Part model, mm, in its own coordinate system. Face numbers are marked on the shaded views. Coordinates: 2 decimals unless noted, no trailing zeros. Loops run counter-clockwise (first coordinate to the right, second up) from the corner with the lowest first, then second, coordinate; pieces in that order, holes last. Notation, with made-up numbers: (41.25, 31) -> (72.25, 31) arc R21 ccw to (72.25, 48) -> close; hole circle Ø2 at (-32, 74). An arc over 180 degrees is marked (long way). Use one line per item in the form item = value. Start each with the question number.
(1) Band-saw the part on B-B on x = -3.75. Give the cut face in (y, z) (3 decimals).
(2) Band-saw the part on A-A on y = 0. Give the cut face in (x, z) (3 decimals), then the cut area to 3 significant figures.
(3) Drill centre lines: L1, parallel to X at y = 22.5, z = 38; L2, parallel to Z at x = -21.5, y = 2.5; L3, parallel to Y at x = -22, z = 3. Where is each one in solid material? Low to high. Write a range as [from, to].
(4) Mould opens along Z. For the marked faces 1, 2 and 3 say: +Z half, -Z half, draft (parallel to the pull), parting line (faces both ways), or undercut.
(5) Band-saw the part on D-D on x = -19. Give the cut face in (y, z) (3 decimals), then the cut area to 3 significant figures.
(6) Pin check, flat tips, straight feed: P1, Ø1, axis at x = -14.5, y = -9.5, coming from the +Z side; P2, Ø10, axis at x = -22.5, y = 13.5, coming from the +Z side; P3, Ø1.5, axis at y = -25.5, z = -22.5, coming from the -X side. Stop position of each tip, or through.
(7) Band-saw the part on C-C on z = 23.5. Give the cut face in (x, y).
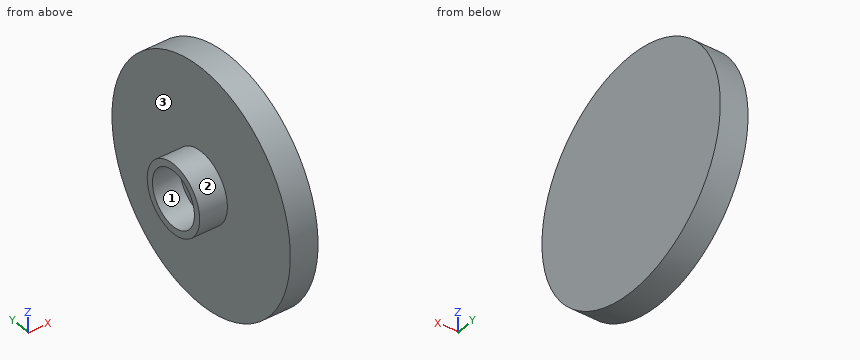
```python
from build123d import *

# Parameters (mm, degrees)
F3_D     = 25.4
F3_DEPTH = 12.701


with BuildPart() as f1:
    # F0 (on Front) → F1 (revolve)
    with BuildSketch(Plane.XZ):
        Polygon((-25.4, 9.525), (0, 9.525), (0, 63.5), (-12.7, 63.5), (-12.7, 25.4), (-25.4, 25.4), align=None)
    revolve(axis=Axis((-12.7, 0, 9.525), (-1, 0, 0)))

    # F3 (through all, one way)
    with BuildSketch(Plane(origin=(-12.7, 0, 0), x_dir=(0, -1, 0), z_dir=(1, 0, 0))):
        with Locations((0, -9.525)):
            Circle(F3_D / 2)
    extrude(amount=-F3_DEPTH, mode=Mode.SUBTRACT)


solid = f1.part
```
A:
q1.outline = circle Ø107.95 at (0, 9.525)
q2.outline = (-25.4, -6.35) -> (-12.7, -6.35) -> (-12.7, -44.45) -> (0, -44.45) -> (0, 63.5) -> (-12.7, 63.5) -> (-12.7, 25.4) -> (-25.4, 25.4) -> (-25.4, 22.225) -> (-12.7, 22.225) -> (-12.7, -3.175) -> (-25.4, -3.175) -> close
q2.area = 1,450 mm²
q3.L1 = [-12.7, 0]
q3.L2 = [-6.15, -2.93], [21.98, 25.2]
q3.L3 = [-14.47, -10.9], [10.9, 14.47]
q4.face_1 = undercut
q4.face_2 = parting line
q4.face_3 = draft
q5.outline = circle Ø31.75 at (0, 9.525); hole circle Ø25.4 at (0, 9.525)
q5.area = 285 mm²
q6.P1 = 22.6
q6.P2 = 22.93
q6.P3 = -12.7
q7.outline = (-25.4, -7.53) -> (-12.7, -7.53) -> (-12.7, -52.13) -> (0, -52.13) -> (0, 52.13) -> (-12.7, 52.13) -> (-12.7, 7.53) -> (-25.4, 7.53) -> close
